For this review, take the finished solid that the model builds, in its own axes (mm). A direction names the side the tool comes from. Give positions to 0.01 mm unless a question says otherwise; leave off trailing zeros. Order: outer loops, then holes, each group sorted by start corner. A loop starts at its lowest first (then second) coordinate and runs counter-clockwise, first axis right, second up. Notation, with made-up numbers: (43, 78) - (94, 78) arc R33 cw to (94, 107) - close; hole circle Ø7 at (81.5, 24). An arc over 180 degrees is marked (long way). One line per item, written item: value.
```python
from build123d import *

# Parameters (mm, degrees)
SKIZZE1_R                            = 9.925
AUFSATZ_LINEAR_AUSTRAGEN1_DEPTH      = 7.15
SKIZZE2_R                            = 12
AUFSATZ_LINEAR_AUSTRAGEN2_DEPTH      = 3
SCHNITT_LINEAR_AUSTRAGEN1_DEPTH      = 21.718892345
SCHNITT_LINEAR_AUSTRAGEN1_DEPTH_BACK = 21.718892345


with BuildPart() as part:
    # Skizze1 → Aufsatz-Linear austragen1 (new body)
    with BuildSketch(Plane(origin=(0, 0, 0), x_dir=(0, 0, -1), z_dir=(1, 0, 0))):
        with Locations((0, 1.5)):
            Circle(SKIZZE1_R)
    extrude(amount=AUFSATZ_LINEAR_AUSTRAGEN1_DEPTH)

    # Skizze2 → Aufsatz-Linear austragen2 (add)
    with BuildSketch(Plane.ZY):
        with Locations((0, 1.5)):
            Circle(SKIZZE2_R)
    extrude(amount=AUFSATZ_LINEAR_AUSTRAGEN2_DEPTH)

    # Skizze3 → Schnitt-Linear austragen1 (cut, two sides: drawn at the far end of the back side and taken through both)
    with BuildSketch(Plane(origin=(7.15, 0, 0), x_dir=(0, 0, -1), z_dir=(1, 0, 0)).offset(-SCHNITT_LINEAR_AUSTRAGEN1_DEPTH_BACK)):
        with BuildLine():
            Line((2.75, -3.04097024), (-2.75, -3.04097024))
            ThreePointArc((-2.75, -3.04097024), (0, 4.1), (2.75, -3.04097024))
        make_face()
    extrude(amount=SCHNITT_LINEAR_AUSTRAGEN1_DEPTH + SCHNITT_LINEAR_AUSTRAGEN1_DEPTH_BACK, mode=Mode.SUBTRACT)


solid = part.part
```
(1) Take a section at B-B (y = 1.5). Write out the cut boundary in (x, z) (3 decimals), then the cut area to 3 significant figures.
Answers below:
outline: (-3, -12) - (0, -12) - (0, -9.925) - (7.15, -9.925) - (7.15, -3.816) - (-3, -3.816) - close; (-3, 3.816) - (7.15, 3.816) - (7.15, 9.925) - (0, 9.925) - (0, 12) - (-3, 12) - close
area: 136 mm^2
(2) Take a section at C-C (z = 8.75). Write out the cut boundary in (x, y), then the cut area to 3 significant figures.
Answers below:
outline: (-3, -6.71) - (0, -6.71) - (0, -3.18) - (7.15, -3.18) - (7.15, 6.18) - (0, 6.18) - (0, 9.71) - (-3, 9.71) - close
area: 116 mm^2
(3) Machinability: for faces 1 (the face through (0, 9, -7)), 2 (the face through (7.15, 4, -2)), which of the approach directions +Z, -Z, +X, -X, +Y, -Y give a long, thin tool a straight path to every point of the face, cutting with its end or side? Answer none if there is none.
Answers below:
face 1: +X
face 2: +Z, -Z, +X, +Y, -Y
(4) Take a section at D-D (y = 6.5). Write out the cut boundary in (x, z).
Answers below:
outline: (-3, -10.91) - (0, -10.91) - (0, -8.57) - (7.15, -8.57) - (7.15, 8.57) - (0, 8.57) - (0, 10.91) - (-3, 10.91) - close
(5) Wall thickness on line 1 (Y direction, x = 4.75, z = 0) (3 decimals); line 2 (Y direction, x = -0.5, z = 0); line 3 (Z direction, x = 0.5, y = 0): over which ranges is each line inside the solid? List them lowest first. Write a range as from..to.
Answers below:
line 1: y = -8.425..-3.041, 4.1..11.425
line 2: y = -10.5..-3.04, 4.1..13.5
line 3: z = -9.81..-4.1, 4.1..9.81
(6) Draft analysis for pull direction Z (two halves, no side actions). For faces 3 (the face through (3.525, -4.539, 7.876)), 4 (the face through (2, 4.1, 0.1)), 5 (the face through (-3, 4.3, -0.2)), 6 (the face through (2, -3.041, 0)), state which applies: pulls with the +Z half, pulls with the -Z half, needs draft (parallel to the pull), parting line crosses it, or undercut.
Answers below:
face 3: parting line crosses it
face 4: undercut
face 5: needs draft
face 6: undercut
(7) For P1, Ø1.5, axis at x = 2.5, z = 3, coming from the +Y side; P2, Ø3, axis at x = 1, z = 1.5, coming from the +Y side; P3, Ø1, axis at y = 0, z = 4, coming from the -X side; P4, Ø2, axis at x = 2.5, y = 3, coming from the +Z side, all flat-tipped, find the tip position at first contact; note any pin that passes through.
Answers below:
P1: stops at y = 11.17
P2: stops at y = 13.49
P3: stops at x = -3
P4: stops at z = 9.91
(8) Take a section at A-A (z = 0). Write out the cut boundary in (x, y) (3 decimals), then the cut area to 3 significant figures.
Answers below:
outline: (-3, -10.5) - (0, -10.5) - (0, -8.425) - (7.15, -8.425) - (7.15, -3.041) - (-3, -3.041) - close; (-3, 4.1) - (7.15, 4.1) - (7.15, 11.425) - (0, 11.425) - (0, 13.5) - (-3, 13.5) - close
area: 141 mm^2
